Geometry check sheet. Reference: drawing and pictorial views, mm from the part's lowest x, y, z. A direction names the side the tool comes from. Give positions to 0.01 mm unless a question says otherwise; leave off trailing zeros. Loops run counter-clockwise (first coordinate to the right, second up) from the corner with the lowest first, then second, coordinate; pieces in that order, holes last. Notation, with made-up numbers: (62, 66.5) - (118, 66.5) arc R35 cw to (118, 102.5) - close; hole circle Ø10 at (56, 76.5). An arc over 180 degrees is marked (long way). Use CSV: the item, a comma, the result in double quotes.
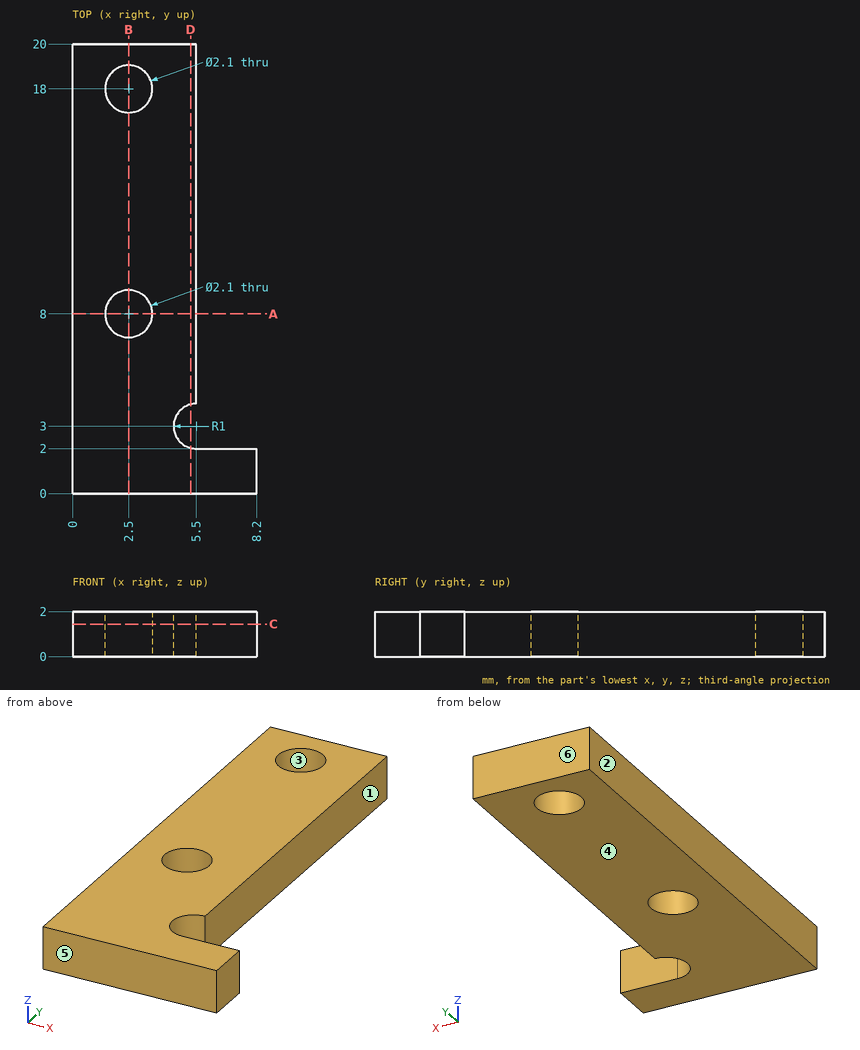
1. Sectioned sample at A-A, the plane y = 8. Record the boundary of the cut face in (x, z), and give its area (3 significant figures).
Completed:
outline,"(0, 0) - (1.45, 0) - (1.45, 2) - (0, 2) - close; (3.55, 0) - (5.5, 0) - (5.5, 2) - (3.55, 2) - close"
area,"6.80 mm²"
2. Release check for a two-part mould opening along Y. For the marked faces 3, 4, 5 and 6 record: released by +Y, released by -Y, zero draft, split by the parting line, or undercut.
Completed:
face 3,"undercut"
face 4,"zero draft"
face 5,"released by -Y"
face 6,"released by +Y"
3. Sectioned sample at D-D, the plane x = 5.25. Record the boundary of the cut face in (y, z), and give its area (3 significant figures).
Completed:
outline,"(0, 0) - (2.03, 0) - (2.03, 2) - (0, 2) - close; (3.97, 0) - (20, 0) - (20, 2) - (3.97, 2) - close"
area,"36.1 mm²"
4. Sectioned sample at C-C, the plane z = 1.45. Record the boundary of the cut face in (x, y), and give its area (3 significant figures).
Completed:
outline,"(0, 0) - (8.2, 0) - (8.2, 2) - (5.5, 2) arc R1 cw to (5.5, 4) - (5.5, 20) - (0, 20) - close; hole circle Ø2.1 at (2.5, 8); hole circle Ø2.1 at (2.5, 18)"
area,"107 mm²"
5. Sectioned sample at B-B, the plane x = 2.5. Record the boundary of the cut face in (y, z).
Completed:
outline,"(0, 0) - (6.95, 0) - (6.95, 2) - (0, 2) - close; (9.05, 0) - (16.95, 0) - (16.95, 2) - (9.05, 2) - close; (19.05, 0) - (20, 0) - (20, 2) - (19.05, 2) - close"
6. Scan lines: line 1 along Y through (x, z) = (2.5, 1.1); line 2 along Y through (x, z) = (2, 1.7); line 3 along X through (y, z) = (16.75, 0.95). Record each from-to range of solid material in increasing order.
Completed:
line 1,"y = 0 to 6.95, 9.05 to 16.95, 19.05 to 20"
line 2,"y = 0 to 7.08, 8.92 to 17.08, 18.92 to 20"
line 3,"x = 0 to 5.5"
7. Set-up check for the marked faces 1 and 2: record each of +Z, -Z, +X, -X, +Y, -Y from which the full face is reachable in a straight line by a thin tool's end or side.
Completed:
face 1,"+Z, -Z, +X, +Y"
face 2,"+Z, -Z, -X, +Y, -Y"
8. Go/stop test with flat-tipped pins: pin 1 Ø2.5 at (x, y) = (2.5, 18) entering from -Z; pin 2 Ø1 at (x, y) = (7, 9.5) entering from +Z. Record where each tip stops, or that it passes through.
Completed:
pin 1,"stops at z = 0"
pin 2,"passes through"
